Can you work these out from the drawing? Everything is in mm from the part's minimum corner. A direction names the side the tool comes from. Round coordinates to 2 decimals unless told otherwise and drop trailing zeros. Loops run counter-clockwise (first coordinate to the right, second up) from the corner with the lowest first, then second, coordinate; pieces in that order, holes last. Notation, with made-up numbers: (75, 47.5) - (90, 47.5) arc R15 cw to (90, 67.5) - close; hole circle Ø11 at (31, 82). An arc over 180 degrees is marked (long way). Answer as a JSON object with one key per item and string values. Group by question number.
1) Will these pins go through, and if not, where does the flat tip stop? P1, Ø2.5, axis at x = 28.59, y = 22, coming from the +Z side; P2, Ø6, axis at y = 15, z = 28, coming from the +X side.
2) Which directions (+Z, -Z, +X, -X, +Y, -Y) give clear straight access to the entire face, cutting with the end or side of a thin tool? Please do the marked faces 1 and 2.
3) I want a section at B-B, the plane x = 28.59. Please give me the cut outline in (y, z), then the cut area to 3 significant figures.
4) I want a section at D-D, the plane z = 35. Give the number of separate pieces and of enclosed holes in the cut face.
5) If I drill on line 1 along Y through (x, z) = (28.59, 1.15); line 2 along Y through (x, z) = (35.59, 1.2); line 3 along X through (y, z) = (14.5, 9), over which ranges is the centre line in solid material (lowest first)? Write a range as [from, to].
6) I want a section at C-C, the plane x = 21.59. Please give me the cut outline in (y, z).
7) I want a section at A-A, the plane z = 10. Please give me the cut outline in (x, y).
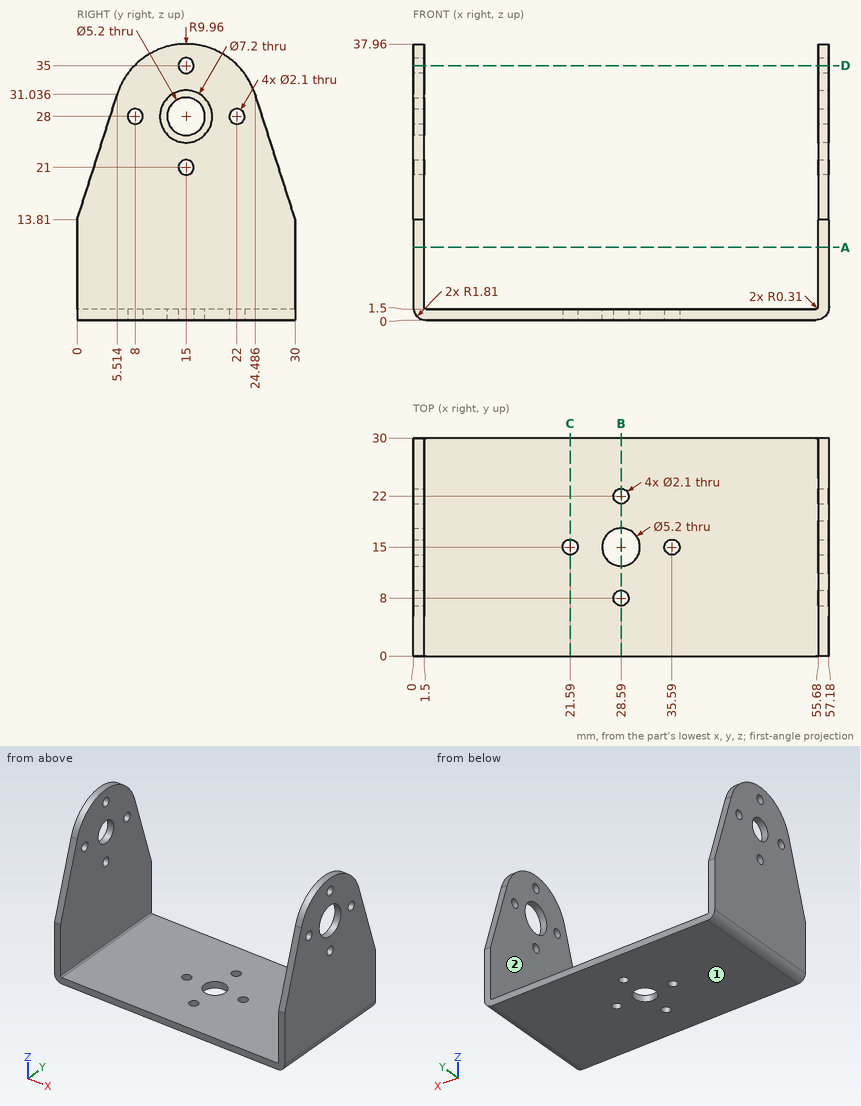
Outcome:
{
 "1": {"P1": "z = 1.5", "P2": "x = 1.5"},
 "2": {"face 1": "-Z, +X, -X, +Y, -Y", "face 2": "+Z, +Y, -Y"},
 "3": {"outline": "(0, 0) - (6.95, 0) - (6.95, 1.5) - (0, 1.5) - close; (9.05, 0) - (12.4, 0) - (12.4, 1.5) - (9.05, 1.5) - close; (17.6, 0) - (20.95, 0) - (20.95, 1.5) - (17.6, 1.5) - close; (23.05, 0) - (30, 0) - (30, 1.5) - (23.05, 1.5) - close", "area": "30.9 mm^2"},
 "4": {"separate pieces": "4", "enclosed holes": "0"},
 "5": {"line 1": "[0, 6.95], [9.05, 12.4], [17.6, 20.95], [23.05, 30]", "line 2": "[0, 13.95], [16.05, 30]", "line 3": "[0, 1.5], [55.68, 57.18]"},
 "6": {"outline": "(0, 0) - (13.95, 0) - (13.95, 1.5) - (0, 1.5) - close; (16.05, 0) - (30, 0) - (30, 1.5) - (16.05, 1.5) - close"},
 "7": {"outline": "(0, 0) - (1.5, 0) - (1.5, 30) - (0, 30) - close; (55.68, 0) - (57.18, 0) - (57.18, 30) - (55.68, 30) - close"}
}
